Check sheet for the modelled part. Datum: model origin and axes. Units: mm. Face numbers are marked on the shaded views. Coordinates: 2 decimals unless noted, no trailing zeros. Write each loop counter-clockwise with the first axis right and the second up, starting at its lowest first coordinate (ties: lowest second). Pieces come first, ordered by that corner, then holes. Notation, with made-up numbers: (33.25, -29.5) - (75.25, -29.5) arc R8 ccw to (75.25, -25.5) - close; hole circle Ø11 at (8, -19.5). An arc over 180 degrees is marked (long way). Answer as CSV lines item,"result". Start each with the question number.
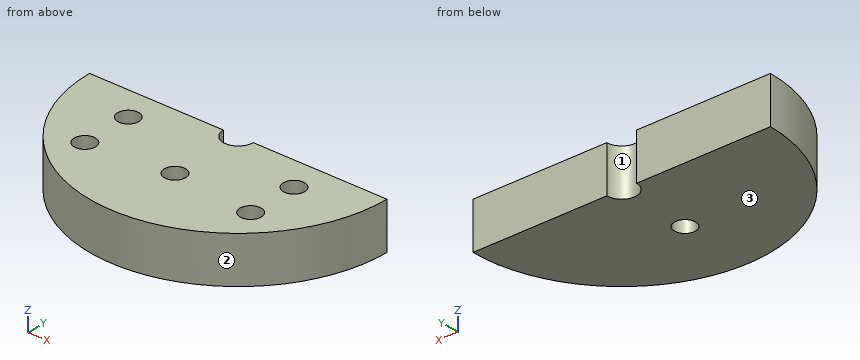
from build123d import *

# Parameters (mm, degrees)
PAD_DEPTH       = 22
SKETCH001_R     = 5
PAD001_DEPTH    = 17
POCKET_DEPTH    = 17
SKETCH002_R     = 5
POCKET001_DEPTH = 22


with BuildPart() as part:
    # Sketch → Pad (new body)
    with BuildSketch(Plane.XY):
        with BuildLine():
            ThreePointArc((-7, 0), (0, -7), (7, 0))
            Line((7, 0), (70, 0))
            ThreePointArc((-70, 0), (0, -70), (70, 0))
            Line((-70, 0), (-7, 0))
        make_face()
    extrude(amount=PAD_DEPTH)

    # Sketch001 (on Face6 of Pad) → Pad001 (join)
    with BuildSketch(Plane.XY.offset(22)):
        with Locations((-39, -39)):
            Circle(SKETCH001_R)
        with Locations((39, -39)):
            Circle(SKETCH001_R)
        with Locations((-39, -15)):
            Circle(SKETCH001_R)
        with Locations((39, -15)):
            Circle(SKETCH001_R)
    extrude(amount=-PAD001_DEPTH)

    # Sketch001 (on Face6 of Pad) → Pocket (cut)
    with BuildSketch(Plane.XY.offset(22)):
        with Locations((-39, -39)):
            Circle(SKETCH001_R)
        with Locations((39, -39)):
            Circle(SKETCH001_R)
        with Locations((-39, -15)):
            Circle(SKETCH001_R)
        with Locations((39, -15)):
            Circle(SKETCH001_R)
    extrude(amount=-POCKET_DEPTH, mode=Mode.SUBTRACT)

    # Sketch002 → Pocket001 (cut)
    with BuildSketch(Plane.XY):
        with Locations((0, -35)):
            Circle(SKETCH002_R)
    extrude(amount=POCKET001_DEPTH, mode=Mode.SUBTRACT)


solid = part.part
(1) Cross-section at D-D on y = -15. Record the boundary of the cut face in (x, z).
(2) Go/stop test with flat-tipped pins: P1, Ø2, axis at x = -50, z = 3, coming from the -Y side; P2, Ø5, axis at y = -19, z = 14.5, coming from the -X side; P3, Ø3, axis at y = -59, z = 8, coming from the +X side. Record where each tip stops, or that it passes through.
(3) Cross-section at B-B on z = 8.25. Record the boundary of the cut face in (x, y).
(4) Release check for a two-part mould opening along X. For the marked faces 1, 2 and 3 record: pulls with the +X half, pulls with the -X half, needs draft (parallel to the pull), parting line crosses it, or undercut.
(5) Material ranges on probe 1 along Y at (x, z) = (39, 11); probe 2 along X at (y, z) = (-12, 19.75); probe 3 along Y at (x, z) = (0, 10.5), recorded low to high. Write a range as from..to.
(6) Cross-section at A-A on x = 0. Record the boundary of the cut face in (y, z), plus the area to 3 significant figures.
(7) Cross-section at C-C on z = 2. Record the boundary of the cut face in (x, y).
Checked values:
1,outline,"(-68.37, 0) - (68.37, 0) - (68.37, 22) - (44, 22) - (44, 5) - (34, 5) - (34, 22) - (-34, 22) - (-34, 5) - (-44, 5) - (-44, 22) - (-68.37, 22) - close"
2,P1,"y = -49.99"
2,P2,"x = -68.03"
2,P3,"x = 39.92"
3,outline,"(-70, 0) arc R70 ccw to (70, 0) - (7, 0) arc R7 cw to (-7, 0) - close; hole circle Ø10 at (-39, -39); hole circle Ø10 at (-39, -15); hole circle Ø10 at (0, -35); hole circle Ø10 at (39, -39); hole circle Ø10 at (39, -15)"
4,face 1,"undercut"
4,face 2,"parting line crosses it"
4,face 3,"needs draft"
5,probe 1,"-58.13..-44, -34..-20, -10..0"
5,probe 2,"-68.96..-43, -35..35, 43..68.96"
5,probe 3,"-70..-40, -30..-7"
6,outline,"(-70, 0) - (-40, 0) - (-40, 22) - (-70, 22) - close; (-30, 0) - (-7, 0) - (-7, 22) - (-30, 22) - close"
6,area,"1,170 mm^2"
7,outline,"(-70, 0) arc R70 ccw to (70, 0) - (7, 0) arc R7 cw to (-7, 0) - close; hole circle Ø10 at (0, -35)"
